```python
from build123d import *

# Parameters (mm, degrees)
SKETCH_1_R      = 10
EXTRUDE_1_DEPTH = 8


with BuildPart() as part:
    # 草图1 → 凸台-拉伸1 (new body)
    with BuildSketch(Plane(origin=(0, 0, 0), x_dir=(1, 0, 0), z_dir=(0, 1, 0))):
        with BuildLine():
            Line((0, -12), (12, -12))
            ThreePointArc((12, -12), (24, 0), (12, 12))
            Line((12, 12), (0, 12))
            ThreePointArc((0, 12), (-12, 0), (0, -12))
        make_face()
        Circle(SKETCH_1_R, mode=Mode.SUBTRACT)
        with BuildLine():
            Line((12, 10), (12, -10))
            ThreePointArc((12, -10), (22, 0), (12, 10))
        make_face(mode=Mode.SUBTRACT)
    extrude(amount=EXTRUDE_1_DEPTH)


solid = part.part
```
Could you check a few things on this model? Use its own coordinates, in mm. A direction names the side the tool comes from. Coordinates: 2 decimals unless noted, no trailing zeros. Loops run counter-clockwise (first coordinate to the right, second up) from the corner with the lowest first, then second, coordinate; pieces in that order, holes last.
1) Imagine slicing it at C-C (x = 15.5). List the corners of the cut face in (y, z) for me, and give its area (3 significant figures).
Reported:
outline: (0, -11.48) - (8, -11.48) - (8, -9.37) - (0, -9.37) - close; (0, 9.37) - (8, 9.37) - (8, 11.48) - (0, 11.48) - close
area: 33.8 mm2
2) Which directions (+Z, -Z, +X, -X, +Y, -Y) give clear straight access to the entire face, cutting with the end or side of a thin tool? Please do faces 1 (the face through (22, 4, 0)), 2 (the face through (6, 4, -12)).
Reported:
face 1: +Y, -Y
face 2: -Z, +X, -X, +Y, -Y
3) Imagine slicing it at B-B (z = -0.5). List the corners of the cut face in (x, y) for me.
Reported:
outline: (-11.99, 0) - (-9.99, 0) - (-9.99, 8) - (-11.99, 8) - close; (9.99, 0) - (12, 0) - (12, 8) - (9.99, 8) - close; (21.99, 0) - (23.99, 0) - (23.99, 8) - (21.99, 8) - close
4) Will this pin go through, and if not, where does the flat tip stop? pin 1 Ø3 at (y, z) = (2, -5.5) entering from -X.
Reported:
pin 1: stops at x = -11.31
5) Thinking about a two-plate mould opening in Z: for faces 3 (the face through (10, 0, -2)), 4 (the face through (6, 4, 12)), 5 (the face through (12, 4, 0)), 6 (the face through (-2.17, 3.94, 9.76)), which applies, released by +Z, released by -Z, zero draft, split by the parting line, or undercut?
Reported:
face 3: zero draft
face 4: released by +Z
face 5: undercut
face 6: undercut
6) Imagine slicing it at D-D (z = -8). List the corners of the cut face in (x, y) for me.
Reported:
outline: (-8.94, 0) - (-6, 0) - (-6, 8) - (-8.94, 8) - close; (6, 0) - (12, 0) - (12, 8) - (6, 8) - close; (18, 0) - (20.94, 0) - (20.94, 8) - (18, 8) - close
7) Please list where these lines run through material, in increasing order: line 1 along X through (y, z) = (4.5, 0.25); line 2 along X through (y, z) = (2.5, -5.5); line 3 along Z through (x, y) = (18, 4.75).
Reported:
line 1: x = -12 to -10, 10 to 12, 22 to 24
line 2: x = -10.67 to -8.35, 8.35 to 12, 20.35 to 22.67
line 3: z = -10.39 to -8, 8 to 10.39
8) Imagine slicing it at A-A (y = 5.75). List the corners of the cut face in (x, z) for me.
Reported:
outline: (0, -12) - (12, -12) arc R12 ccw to (12, 12) - (0, 12) arc R12 ccw to start; hole circle Ø20 at (0, 0); hole (12, -10) arc R10 ccw to (12, 10) - close
